For this review, take the finished solid that the model builds, in its own axes (mm). Give positions to 0.01 mm unless a question says otherwise; leave off trailing zeros. Write each loop counter-clockwise with the first axis right and the second up, starting at its lowest first coordinate (ties: lowest second). Pieces come first, ordered by that corner, then holes.
Q1. For line 1 (X direction, y = -0.8, z = -69.85); line 2 (X direction, y = -0.8, z = 105.41); line 3 (Z direction, x = 26.5, y = -0.9), list the stretches that pass through material, from the lowest coordinate up.
Q2. Insertion check: P1, Ø2.5, axis at x = -54.77, z = 105.41, coming from the +Y side. The pin has a flat end and moves straight along its axis. Give the tip position at first contact, or say it passes through.
Q3. We need section A-A (y = -1.05). Give the number of separate pieces and of enclosed holes in the cut face, then the cut area to 3 significant figures.
Q4. We need section B-B (x = -44). Write out the cut boundary in (y, z), then the cut area to 3 significant figures.
Q5. We need section C-C (x = 10.5). Write out the cut boundary in (y, z), then the cut area to 3 significant figures.
```python
from build123d import *

# Parameters (mm, degrees)
SKETCH1_W                     = 130.175
SKETCH1_H                     = 914.4
BOSS_EXTRUDE1_DEPTH           = 1.5875
SKETCH2_R                     = 1.5875
SKETCH2_R_2                   = 3.175
CUT_EXTRUDE2_DEPTH            = 462.812454155
SKETCH3_R                     = 1.5875
CUT_EXTRUDE3_DEPTH            = 462.812454155
STRUTMOUNTINGHOLES_DEPTH      = 462.812454155
STRUTMOUNTINGHOLES_DEPTH_BACK = 462.812454155
SKETCH5_R                     = 1.5875


with BuildPart() as part:
    # Sketch1 → Boss-Extrude1 (new body)
    with BuildSketch(Plane(origin=(0, 0, 0), x_dir=(1, 0, 0), z_dir=(0, 1, 0))):
        Rectangle(SKETCH1_W, SKETCH1_H)
    extrude(amount=-BOSS_EXTRUDE1_DEPTH)

    # Sketch2 → Cut-Extrude2 (cut, through all)
    with BuildSketch(Plane(origin=(0, 0, 0), x_dir=(1, 0, 0), z_dir=(0, 1, 0))):
        with Locations(Location((54.76875, -447.675, 0), (0, 0, 270))):
            Circle(SKETCH2_R)
        with Locations(Location((54.76875, -311.15, 0), (0, 0, 270))):
            Circle(SKETCH2_R_2)
        with Locations(Location((54.76875, 447.675, 0), (0, 0, 270))):
            Circle(SKETCH2_R)
        with Locations(Location((54.76875, 69.85, 0), (0, 0, 270))):
            Circle(SKETCH2_R_2)
        with Locations(Location((54.76875, 295.275, 0), (0, 0, 270))):
            Circle(SKETCH2_R)
    cut_extrude2 = extrude(amount=-CUT_EXTRUDE2_DEPTH, mode=Mode.SUBTRACT)

    # Mirror2: Cut-Extrude2 across plane
    add(cut_extrude2.mirror(Plane.ZY), mode=Mode.SUBTRACT)

    # Sketch3 → Cut-Extrude3 (cut, through all)
    with BuildSketch(Plane.XZ.offset(1.5875)):
        Polygon((-65.0875, -457.2), (46.0375, -457.2), (-65.0875, -304.8), align=None)
        with Locations((-54.76875, -447.675)):
            Circle(SKETCH3_R, mode=Mode.SUBTRACT)
    extrude(amount=-CUT_EXTRUDE3_DEPTH, mode=Mode.SUBTRACT)

    # Sketch5 → StrutMountingHoles (cut, two sides: drawn at the far end of the back side and taken through both)
    with BuildSketch(Plane(origin=(0, -1.5875, 0), x_dir=(-1, 0, 0), z_dir=(0, -1, 0)).offset(-STRUTMOUNTINGHOLES_DEPTH_BACK)):
        with Locations(Location((54.76875, -123.19, 0), (0, 0, 90))):
            Circle(SKETCH5_R)
        with Locations(Location((54.76875, -105.41, 0), (0, 0, 90))):
            Circle(SKETCH5_R)
    extrude(amount=STRUTMOUNTINGHOLES_DEPTH + STRUTMOUNTINGHOLES_DEPTH_BACK, mode=Mode.SUBTRACT)


solid = part.part
```
Computed:
1. line 1: x = -65.09 to -57.94, -51.59 to 51.59, 57.94 to 65.09
1. line 2: x = -65.09 to -56.36, -53.18 to 65.09
1. line 3: z = -430.41 to 457.2
2. P1: passes through
3. separate pieces: 1
3. enclosed holes: 11
3. area: 110,000 mm2
4. outline: (-1.59, -333.72) - (0, -333.72) - (0, 457.2) - (-1.59, 457.2) - close
4. area: 1,260 mm2
5. outline: (-1.59, -408.46) - (0, -408.46) - (0, 457.2) - (-1.59, 457.2) - close
5. area: 1,370 mm2
